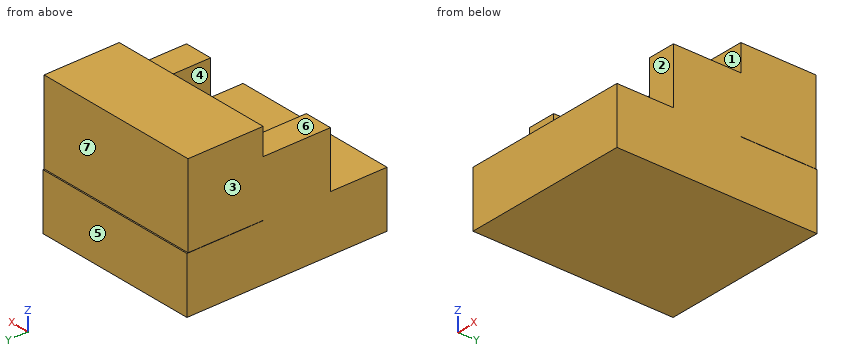
```python
from build123d import *

# Parameters (mm, degrees)
F0_W     = 75.78361
F0_H     = 90.648856
F1_DEPTH = 25.4
F2_W     = 12.7
F2_H     = 30.48
F3_DEPTH = 50.8
F4_W     = 75.78361
F4_H     = 37.308857
F5_DEPTH = 34.036


with BuildPart() as f1:
    # F0 (on Top) → F1 (new body)
    with BuildSketch(Plane.XY):
        with Locations((1.457378, -10.784591)):
            Rectangle(F0_W, F0_H)
    extrude(amount=F1_DEPTH)

    # F2 (on Top) → F3 (join)
    with BuildSketch(Plane.XY):
        with Locations((-30.084427, -15.24)):
            Rectangle(F2_W, F2_H)
        with Locations((32.999183, -15.24)):
            Rectangle(F2_W, F2_H)
    extrude(amount=F3_DEPTH)

    # F4 (on Front) → F5 (join)
    with BuildSketch(Plane.XZ):
        with Locations((1.457378, 44.158525)):
            Rectangle(F4_W, F4_H)
    extrude(amount=-F5_DEPTH)


solid = f1.part
```
Could you check a few things on this model? Use its own coordinates, in mm. Face numbers are marked on the shaded views. A direction names the side the tool comes from. Round coordinates to 2 decimals unless told otherwise and drop trailing zeros. Loops run counter-clockwise (first coordinate to the right, second up) from the corner with the lowest first, then second, coordinate; pieces in that order, holes last. Notation, with made-up numbers: M 56.25,-37.75 L 104.25,-37.75 A9 cw 104.25,-32.75 Z; hole C 79.5,71.25 d10. An arc over 180 degrees is marked long. Answer as CSV lines item,"result".
1) Imagine slicing it at D-D on z = 29.5. List the corners of the cut face in (x, y) for me.
From the geometry:
outline,"M -36.43,-30.48 L -23.73,-30.48 L -23.73,0 L 26.65,0 L 26.65,-30.48 L 39.35,-30.48 L 39.35,34.04 L -36.43,34.04 Z"
2) Imagine slicing it at B-B on y = -28. List the corners of the cut face in (x, z) for me, and give its area (3 significant figures).
From the geometry:
outline,"M -36.43,0 L 39.35,0 L 39.35,50.8 L 26.65,50.8 L 26.65,25.4 L -23.73,25.4 L -23.73,50.8 L -36.43,50.8 Z"
area,"2,570 mm^2"
3) If I drill on probe 1 along X at (y, z) = (-19, 45.5); probe 2 along Z at (x, y) = (14, -10.5); probe 3 along Y at (x, z) = (1, 40), over which ranges is the centre line in solid material (lowest first)?
From the geometry:
probe 1,"-36.43 to -23.73, 26.65 to 39.35"
probe 2,"0 to 25.4"
probe 3,"0 to 34.04"
4) We'd pull the mould along X, two halves only. Please class the marked faces 1, 2 and 3: released by +X, released by -X, zero draft, split by the parting line, or undercut.
From the geometry:
face 1,"undercut"
face 2,"zero draft"
face 3,"released by -X"
5) Which directions (+Z, -Z, +X, -X, +Y, -Y) give clear straight access to the entire face, cutting with the end or side of a thin tool? Please do the marked faces 4, 5, 6 and 7.
From the geometry:
face 4,"+Z, -Y"
face 5,"+Z, -Z, +X, -X, +Y"
face 6,"+Z, +X, -X, -Y"
face 7,"+Z, +X, -X, +Y"
6) Imagine slicing it at A-A on x = -7.5. List the corners of the cut face in (y, z) for me.
From the geometry:
outline,"M -56.11,0 L 34.54,0 L 34.54,25.4 L -56.11,25.4 Z; M 0,25.5 L 34.04,25.5 L 34.04,62.81 L 0,62.81 Z"
7) Imagine slicing it at C-C on x = -29.5. List the corners of the cut face in (y, z) for me.
From the geometry:
outline,"M -56.11,0 L 34.54,0 L 34.54,25.4 L 0,25.4 L 0,25.5 L 34.04,25.5 L 34.04,62.81 L 0,62.81 L 0,50.8 L -30.48,50.8 L -30.48,25.4 L -56.11,25.4 Z"
8) For pin 1 Ø4 at (x, z) = (-31.5, 33) entering from -Y; pin 2 Ø11 at (x, z) = (12, 48) entering from +Y; pin 3 Ø1.5 at (x, y) = (27.5, -3.5) entering from +Z, each with a flat end and sliding along its axis, tell me the tip position at first contact or that it passes through.
From the geometry:
pin 1,"y = -30.48"
pin 2,"y = 34.04"
pin 3,"z = 50.8"
